Input: part model. Units: mm. Frame: model coordinates. A direction names the side the tool comes from. Round coordinates to 2 decimals unless told otherwise and drop trailing zeros. Loops run counter-clockwise (first coordinate to the right, second up) from the corner with the lowest first, then second, coordinate; pieces in that order, holes last.
1) Ray query, line 1 along Y through (x, z) = (0, 3.25) (1 decimal); line 2 along X through (y, z) = (-116, 3.5); line 3 along Y through (x, z) = (-1, 2.5). Return the intervals inside material, ascending.
2) Section A-A, the plane z = 4.25. State how many separate pieces and enclosed holes the cut face has, and give its area (3 significant figures).
3) Access query for faces 1 (the face through (7.98, -4.33, 3.13)), 2 (the face through (22.86, -60, 3)), 3 (the face through (14.75, -118.95, 3.13)). Directions: +Z, -Z, +X, -X, +Y, -Y. A direction counts if a zero-diameter tool reaches every point of the face in a straight line with its end or side. Return the directions, or none.
4) Section D-D, the plane y = -78. Return loops of the section in (x, z).
5) First-contact query: pin 1 (1.5 mm diameter, centred on x = 15, z = 4, fed in from +Y); pin 2 (3 mm diameter, centred on x = 10, z = 3, fed in from +Y); pin 3 (10.5 mm diameter, centred on x = 0, y = 0, fed in from +Z); pin 4 (3 mm diameter, centred on y = -18.5, z = 4, fed in from -X). Flat tips, straight axial feed; report the tip coordinate or a pass-through.
6) Draft query along X for faces 4 (the face through (18.78, -135.25, 3.13)), 5 (the face through (8.05, 4.3, 3.13)), 6 (the face through (14.476, -4.534, 3.131)), 7 (the face through (14, 3.81, 3)). Return one class per face: pulls with the +X half, pulls with the -X half, needs draft (parallel to the pull), parting line crosses it, or undercut.
from build123d import *

# Parameters (mm, degrees)
ESQUISSE1_R        = 6.4135
BOSS_EXTRU_1_DEPTH = 6.35


with BuildPart() as part:
    # Esquisse1 → Boss.-Extru.1 (new body)
    with BuildSketch(Plane(origin=(154.130652136, 0, 0), x_dir=(1, 0, 0), z_dir=(0, 0, 1))):
        with BuildLine():
            Line((-138.890652136, -6.35), (-138.890652136, -116.508078107))
            ThreePointArc((-138.890652136, -116.508078107), (-139.393732658, -118.985179762), (-140.823260832, -121.069783278))
            ThreePointArc((-140.823260832, -121.069783278), (-135.080652136, -135.255), (-129.338043441, -121.069783278))
            ThreePointArc((-129.338043441, -121.069783278), (-130.767571615, -118.985179762), (-131.270652136, -116.508078107))
            Line((-131.270652136, -116.508078107), (-131.270652136, -2.54))
            ThreePointArc((-131.270652136, -2.54), (-133.130524076, 1.950128061), (-137.620652136, 3.81))
            Line((-137.620652136, 3.81), (-143.638730244, 3.81))
            ThreePointArc((-143.638730244, 3.81), (-146.115831899, 4.313080521), (-148.200435415, 5.742608696))
            ThreePointArc((-148.200435415, 5.742608696), (-162.385652136, 0), (-148.200435415, -5.742608696))
            ThreePointArc((-148.200435415, -5.742608696), (-146.115831899, -4.313080521), (-143.638730244, -3.81))
            Line((-143.638730244, -3.81), (-141.430652136, -3.81))
            ThreePointArc((-141.430652136, -3.81), (-139.634600912, -4.553948776), (-138.890652136, -6.35))
        make_face()
        with Locations((-135.080652136, -127)):
            Circle(ESQUISSE1_R, mode=Mode.SUBTRACT)
        with Locations((-154.130652136, 0)):
            Circle(ESQUISSE1_R, mode=Mode.SUBTRACT)
    extrude(amount=BOSS_EXTRU_1_DEPTH)


solid = part.part
Final values:
1. line 1: y = -8.3 to -6.4, 6.4 to 8.3
1. line 2: x = 15.24 to 22.86
1. line 3: y = -8.19 to -6.34, 6.34 to 8.19
2. separate pieces: 1
2. enclosed holes: 2
2. area: 1,160 mm2
3. face 1: +Z, -Z, -Y
3. face 2: +Z, -Z, +X, +Y
3. face 3: +Z, -Z, -X
4. outline: (15.24, 0) - (22.86, 0) - (22.86, 6.35) - (15.24, 6.35) - close
5. pin 1: stops at y = 3.81
5. pin 2: stops at y = 4.13
5. pin 3: passes through
5. pin 4: stops at x = 15.24
6. face 4: parting line crosses it
6. face 5: pulls with the +X half
6. face 6: undercut
6. face 7: needs draft
